Work out the finished part from the listing and answer in its coordinate system (mm). Face numbers are marked on the shaded views. A direction names the side the tool comes from. Give positions to 0.01 mm unless a question says otherwise; leave off trailing zeros. Write each loop counter-clockwise with the first axis right and the second up, starting at its lowest first coordinate (ties: lowest second). Pieces come first, ordered by that corner, then holes.
1) Find section C-C (z = 20). Determine the outline of the cut face in (x, y), plus the area to 3 significant figures.
2) Find section A-A (y = -44.5). Determine the outline of the cut face in (x, z).
3) Straight lines are drawn through the part: probe 1 along X at (y, z) = (-59.5, 28.25); probe 2 along X at (y, z) = (13, 4.5); probe 3 along Y at (x, z) = (15, 28.75). For each, find the intervals that lie inside material, in ascending order.
4) A tool of negligible diameter and unlimited length cuts with its end or side. For the marked faces 4, 5 and 6, from which of +Z, -Z, +X, -X, +Y, -Y can it reach the whole face along a straight path? Write none if from no direction.
5) Given pin 1 Ø1.5 at (y, z) = (-69, 28) entering from +X; pin 2 Ø2.5 at (x, y) = (-34.81, -25.27) entering from -Z; pin 3 Ø2.5 at (x, z) = (-44, 28.5) entering from -Y; pin 4 Ø8 at (y, z) = (-60.5, 26) entering from -X, each flat-ended and moving along its own axis, determine where each tip first touches the part or whether it passes through.
6) Find section B-B (y = -2). Determine the outline of the cut face in (x, z), plus the area to 3 significant figures.
7) Find section D-D (x = 0). Determine the outline of the cut face in (y, z).
8) Determine the mould class of the marked faces 1, 2 and 3 for opening direction X: pulls with the +X half, pulls with the -X half, needs draft (parallel to the pull), parting line crosses it, or undercut.
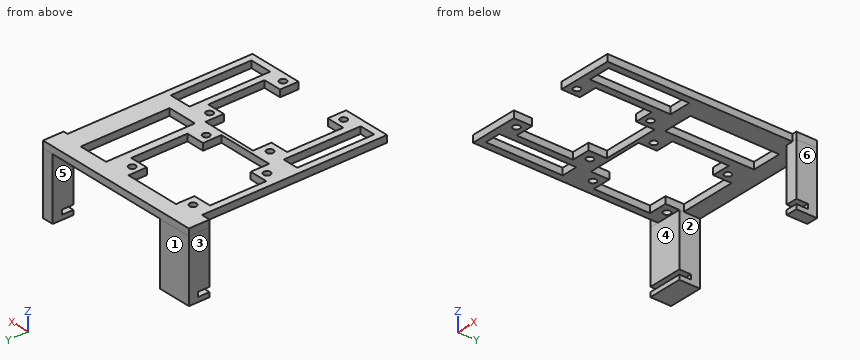
```python
from build123d import *

# Parameters (mm, degrees)
CROQUIS1_W                = 5
CROQUIS1_H                = 9
SALIENTE_EXTRUIR1_DEPTH   = 27
CROQUIS1_W_2              = 14.88
SALIENTE_EXTRUIR1_2_DEPTH = 27
CROQUIS2_R                = 1.5
CROQUIS2_W                = 9.622736673
CROQUIS2_H                = 35.115677267
CROQUIS2_W_2              = 7
CROQUIS2_H_2              = 33.5
CROQUIS2_W_3              = 13
CROQUIS2_H_3              = 38.689553843
SALIENTE_EXTRUIR2_DEPTH   = 3
CORTAR_EXTRUIR1_START     = -75
CROQUIS3_W                = 2
CROQUIS3_H                = 5
CORTAR_EXTRUIR1_DEPTH     = 75


with BuildPart() as part:
    # Croquis1 → Saliente-Extruir1 (new body)
    with BuildSketch(Plane.XY):
        with Locations((27.073193316, 13.235294118)):
            Rectangle(CROQUIS1_W, CROQUIS1_H)
    extrude(amount=SALIENTE_EXTRUIR1_DEPTH)



with BuildPart() as body_2:
    # Croquis1 → Saliente-Extruir1 2 (new body)
    with BuildSketch(Plane.XY):
        with Locations((-37.986806684, 13.235294118)):
            Rectangle(CROQUIS1_W_2, CROQUIS1_H)
    extrude(amount=SALIENTE_EXTRUIR1_2_DEPTH)


with BuildPart() as part_1:
    add(part.part)

    add(body_2.part)  # Saliente-Extruir2 merges body 2
    # Croquis2 → Saliente-Extruir2 (add)
    with BuildSketch(Plane.XY.offset(27)):
        Polygon((-45.425929091, 8.73433808), (-41.548665764, 8.73433808), (-41.548665764, -71.76566192), (-28.548665764, -71.76566192), (-20.548665764, -71.76566192), (-20.548665764, -63.76566192), (-28.548665764, -63.76566192), (-28.548665764, -39.26566192), (-20.548665764, -39.26566192), (-20.548665764, -31.26566192), (3.951334236, -31.26566192), (3.951334236, -39.26566192), (11.951334236, -39.26566192), (11.951334236, -63.76566192), (3.951334236, -63.76566192), (3.951334236, -71.745971947), (15.951334236, -71.745971947), (27.574070909, -71.745971947), (27.574070909, 8.73433808), (29.574070909, 8.73433808), (29.573193316, 17.735294118), (-45.425929091, 17.73433808), align=None)
        with Locations((-24.548665764, -35.26566192)):
            Circle(CROQUIS2_R, mode=Mode.SUBTRACT)
        with Locations((7.451334236, -36.017200949)):
            Circle(CROQUIS2_R, mode=Mode.SUBTRACT)
        with Locations((-24.548665764, -67.26566192)):
            Circle(CROQUIS2_R, mode=Mode.SUBTRACT)
        with Locations((7.451334236, -68.017200949)):
            Circle(CROQUIS2_R, mode=Mode.SUBTRACT)
        with Locations((-34.548665764, 6.73433808)):
            Circle(CROQUIS2_R, mode=Mode.SUBTRACT)
        with Locations((-34.806623414, -25.26566192)):
            Circle(CROQUIS2_R, mode=Mode.SUBTRACT)
        with Locations((-2.806623414, -25.892139455)):
            Circle(CROQUIS2_R, mode=Mode.SUBTRACT)
        with Locations((-2.548665764, 6.107860545)):
            Circle(CROQUIS2_R, mode=Mode.SUBTRACT)
        Polygon((-30.548665764, -29.76566192), (-30.548665764, -21.76566192), (-38.548665764, -21.76566192), (-38.548665764, 2.73433808), (-30.548665764, 2.73433808), (-30.548665764, 10.73433808), (-6.048665764, 10.73433808), (-6.048665764, 2.73433808), (1.951334236, 2.73433808), (1.951334236, -21.76566192), (-6.048665764, -21.76566192), (-6.048665764, -29.76566192), align=None, mode=Mode.SUBTRACT)
        with Locations((19.762702573, -51.188133314)):
            Rectangle(CROQUIS2_W, CROQUIS2_H, mode=Mode.SUBTRACT)
        with Locations((-35.048665764, -52.01566192)):
            Rectangle(CROQUIS2_W_2, CROQUIS2_H_2, mode=Mode.SUBTRACT)
        with Locations((11.951334236, -8.610438842)):
            Rectangle(CROQUIS2_W_3, CROQUIS2_H_3, mode=Mode.SUBTRACT)
    extrude(amount=SALIENTE_EXTRUIR2_DEPTH)

    # Croquis3 → Cortar-Extruir1 (cut)
    with BuildSketch(Plane(origin=(29.573193316, 0, 0), x_dir=(0, 0, -1), z_dir=(1, 0, 0)).offset(CORTAR_EXTRUIR1_START)):
        with Locations((-3, 11.235294118)):
            Rectangle(CROQUIS3_W, CROQUIS3_H)
    extrude(amount=CORTAR_EXTRUIR1_DEPTH, mode=Mode.SUBTRACT)


solid = part_1.part
```
Results:
1. outline: (-45.43, 8.74) - (-30.55, 8.74) - (-30.55, 17.74) - (-45.43, 17.74) - close; (24.57, 8.74) - (29.57, 8.74) - (29.57, 17.74) - (24.57, 17.74) - close
1. area: 179 mm2
2. outline: (-41.55, 27) - (-38.55, 27) - (-38.55, 30) - (-41.55, 30) - close; (-31.55, 27) - (-28.55, 27) - (-28.55, 30) - (-31.55, 30) - close; (11.95, 27) - (14.95, 27) - (14.95, 30) - (11.95, 30) - close; (24.57, 27) - (27.57, 27) - (27.57, 30) - (24.57, 30) - close
3. probe 1: x = -41.55 to -38.55, -31.55 to -28.55, 11.95 to 14.95, 24.57 to 27.57
3. probe 2: x = -45.43 to -30.55, 24.57 to 29.57
3. probe 3: y = -71.75 to -68.75, -33.63 to -27.96, 10.73 to 17.74
4. face 4: -Z, +X, -X, -Y
4. face 5: -Z, +Y, -Y
4. face 6: +Z, -Z, +X, +Y, -Y
5. pin 1: stops at x = 27.57
5. pin 2: passes through
5. pin 3: stops at y = 8.73
5. pin 4: stops at x = -41.55
6. outline: (-41.55, 27) - (-38.55, 27) - (-38.55, 30) - (-41.55, 30) - close; (1.95, 27) - (5.45, 27) - (5.45, 30) - (1.95, 30) - close; (18.45, 27) - (27.57, 27) - (27.57, 30) - (18.45, 30) - close
6. area: 46.9 mm2
7. outline: (-31.27, 27) - (-21.77, 27) - (-21.77, 30) - (-31.27, 30) - close; (2.73, 27) - (17.73, 27) - (17.73, 30) - (2.73, 30) - close
8. face 1: needs draft
8. face 2: undercut
8. face 3: pulls with the -X half
